```python
from build123d import *

# Parameters (mm, degrees)
SKETCH1_W           = 63.5
SKETCH1_H           = 19.05
SKETCH1_R           = 4.7625
SKETCH1_R_2         = 3.9878
BOSS_EXTRUDE1_DEPTH = 25.4
SKETCH2_R           = 2
CUT_EXTRUDE1_DEPTH  = 6.35


with BuildPart() as part:
    # Sketch1 → Boss-Extrude1 (new body)
    with BuildSketch(Plane.XY):
        Rectangle(SKETCH1_W, SKETCH1_H)
        Circle(SKETCH1_R, mode=Mode.SUBTRACT)
        with Locations((-22.225, -3.175)):
            Circle(SKETCH1_R_2, mode=Mode.SUBTRACT)
        with Locations((22.225, -3.175)):
            Circle(SKETCH1_R_2, mode=Mode.SUBTRACT)
    extrude(amount=-BOSS_EXTRUDE1_DEPTH)

    # Sketch2 → Cut-Extrude1 (cut)
    with BuildSketch(Plane.ZY.offset(31.75)):
        with Locations((-12.7, 3.175)):
            Circle(SKETCH2_R)
    cut_extrude1 = extrude(amount=-CUT_EXTRUDE1_DEPTH, mode=Mode.SUBTRACT)

    # Mirror1: Cut-Extrude1 across plane
    add(cut_extrude1.mirror(Plane.ZY), mode=Mode.SUBTRACT)


solid = part.part
```
Source: CAD feature listing. Evaluate the final solid. Frame: model axes, mm. A direction names the side the tool comes from. Round coordinates to 2 decimals unless told otherwise and drop trailing zeros. Order: outer loops, then holes, each group sorted by start corner. A loop starts at its lowest first (then second) coordinate and runs counter-clockwise, first axis right, second up. Notation, with made-up numbers: (46, -17) -> (102, -17) arc R36 cw to (102, 22) -> close; hole circle Ø1 at (-23.5, -3.75). An arc over 180 degrees is marked (long way). One line per item, written item: value. Start each with the question number.
Q1. Access query for faces 1 (the cylindrical face through (-28.6, 3.8, -10.8)), 2 (the cylindrical face through (19.06, -5.6, -12.52)), 3 (the cylindrical face through (28.6, 3.8, -10.8)). Directions: +Z, -Z, +X, -X, +Y, -Y. A direction counts if a zero-diameter tool reaches every point of the face in a straight line with its end or side. Return the directions, or none.
Q2. Section query A-A (x = 0). Return the cut outline in (y, z) (1 decimal), plus the area to 3 significant figures.
Q3. Pin query (flat end, axial travel): pin 1 (6.5 mm diameter, centred on x = -22.225, y = -3.175, fed in from +Z); pin 2 (2 mm diameter, centred on y = 3, z = -13, fed in from +X); pin 3 (2 mm diameter, centred on y = 3, z = -12, fed in from -X). Return the tip coordinate at first contact, or that it passes through.
Q4. Material intervals for probe 1 along Y at (x, z) = (0, -12.25) (1 decimal); probe 2 along X at (y, z) = (0.5, -15); probe 3 along Y at (x, z) = (-28.75, -12.7) (3 decimals), sorted ascending.
Q5. Section query C-C (z = -21.25). Give the number of separate pieces and of enclosed holes in the cut face, plus the area to 3 significant figures.
Q6. Section query B-B (y = 2). Return the cut outline in (x, z), plus the area to 3 significant figures.
Q7. Draft query along Y for faces 4 (the flat face through (0, -9.525, -13)), 5 (the cylindrical face through (-3.78, -2.9, -12.52)), 6 (the flat face through (31.75, 0, -13)). Return one class per face: pulls with the +Y half, pulls with the -Y half, needs draft (parallel to the pull), parting line crosses it, or undercut.
Q8. Section query D-D (x = -24). Return the cut outline in (y, z) (3 decimals), plus the area to 3 significant figures.
Findings below:
1. face 1: -X
1. face 2: +Z, -Z
1. face 3: +X
2. outline: (-9.5, -25.4) -> (-4.8, -25.4) -> (-4.8, 0) -> (-9.5, 0) -> close; (4.8, -25.4) -> (9.5, -25.4) -> (9.5, 0) -> (4.8, 0) -> close
2. area: 242 mm²
3. pin 1: through
3. pin 2: x = 25.4
3. pin 3: x = -25.4
4. probe 1: -9.5 to -4.8, 4.8 to 9.5
4. probe 2: -31.75 to -23.77, -20.68 to -4.74, 4.74 to 20.68, 23.77 to 31.75
4. probe 3: -9.525 to 1.175, 5.175 to 9.525
5. separate pieces: 1
5. enclosed holes: 3
5. area: 1,040 mm²
6. outline: (-31.75, -25.4) -> (-4.32, -25.4) -> (-4.32, 0) -> (-31.75, 0) -> (-31.75, -11.08) -> (-25.4, -11.08) -> (-25.4, -14.32) -> (-31.75, -14.32) -> close; (4.32, -25.4) -> (31.75, -25.4) -> (31.75, -14.32) -> (25.4, -14.32) -> (25.4, -11.08) -> (31.75, -11.08) -> (31.75, 0) -> (4.32, 0) -> close
6. area: 1,350 mm²
7. face 4: pulls with the -Y half
7. face 5: undercut
7. face 6: needs draft
8. outline: (-9.525, -25.4) -> (-6.746, -25.4) -> (-6.746, 0) -> (-9.525, 0) -> close; (0.396, -25.4) -> (9.525, -25.4) -> (9.525, 0) -> (0.396, 0) -> close
8. area: 302 mm²
